Geometry: final body of the model. Coordinates: model frame, mm. A direction names the side the tool comes from. Coordinates: 2 decimals unless noted, no trailing zeros. Write each loop counter-clockwise with the first axis right and the second up, starting at its lowest first coordinate (ties: lowest second). Pieces come first, ordered by that corner, then holes. Notation, with made-up numbers: M 47,39.25 L 82,39.25 A17 ccw 82,71.25 Z; hole C 64,44 d1. An arc over 180 degrees is marked long. Write item = value, one per line. Start each with the question number.
Item 1: Pull-direction query (X, two-part tool) for faces 1 (the flat face through (-18.492, -4, 3)), 2 (the flat face through (25.4, -8, 3)), 3 (the cylindrical face through (12.532, -13.154, 3.026)), 4 (the flat face through (-24, -24.724, 3)); classes: +X half, -X half, draft (parallel to the pull), parting line (faces both ways), or undercut.
Item 2: Section B-B on y = 0.15. Output: boundary loops of the cut face in (x, z).
Item 3: Reachability of faces 5 (the flat face through (24, -5.84, 3)), 6 (the flat face through (-21, -1.039, 3)), 7 (the flat face through (-17.64, -19.01, 2.94)), 8 (the flat face through (-28, -10.437, 3)) from +Z, -Z, +X, -X, +Y, -Y: full face, straight path, thin tool, end or side. Return the list, or none.
Item 4: Section C-C on z = 0.9. Give the number of separate pieces and of enclosed holes in the cut face, plus the area to 3 significant figures.
Item 5: Section D-D on y = -17. Output: boundary loops of the cut face in (x, z).
Item 6: Ray query, L1, parallel to X at y = -1.5, z = 1.95 (3 decimals); L2, parallel to Y at x = -26, z = 1.85; L3, parallel to Y at x = 0.5, z = 2.6. Return the intervals inside material, ascending. Write a range as [from, to].
Item 7: First-contact query: pin 1 Ø1.4 at (y, z) = (-2, 1.5) entering from -X; pin 2 Ø3 at (y, z) = (-4, 4.5) entering from -X; pin 3 Ø0.6 at (x, z) = (-19, 2.5) entering from +Y. Flat tips, straight axial feed; report the tip coordinate or a pass-through.
Item 8: Section A-A on x = -1.5. Output: boundary loops of the cut face in (y, z).
from build123d import *

# Parameters (mm, degrees)
SKETCH1_W           = 12.3904
SKETCH1_H           = 13
BOSS_EXTRUDE1_DEPTH = 5.969
CUT_EXTRUDE1_DEPTH  = 41.286380146
SKETCH3_R           = 0.1984375
CUT_EXTRUDE2_DEPTH  = 41.286380146
FILLET1_R           = 3.175
FILLET2_R           = 1.5875
SKETCH4_W           = 12.7
SKETCH4_H           = 11.1125
CUT_EXTRUDE3_DEPTH  = 41.286380146
SKETCH5_W           = 10.16
SKETCH5_H           = 0.5
CUT_EXTRUDE4_DEPTH  = 41.286380146
FILLET8_R           = 0.1
CUT_EXTRUDE5_DEPTH  = 41.286380146
FILLET9_R           = 6.35


with BuildPart() as part:
    # Sketch1 → Boss-Extrude1 (new body)
    with BuildSketch(Plane.XY):
        Polygon((25.4, 2.263), (25.4, -10.437), (31.242, -10.437), (31.242, -23.137), (25.4, -23.137), (25.4, -24.7245), (22.225, -24.7245), (12.7, -12.85), (-12.7, -12.85), (-22.225, -24.7245), (-25.4, -24.7245), (-25.4, -23.137), (-31.242, -23.137), (-31.242, -10.437), (-25.4, -10.437), (-25.4, 2.263), (-31.242, 2.263), (-31.242, 14.963), (-25.4, 14.963), (-25.4, 18.138), (-22.225, 18.138), (-12.7, 12.85), (12.7, 12.85), (22.225, 18.138), (25.4, 18.138), (25.4, 14.963), (31.242, 14.963), (31.242, 2.263), align=None)
        Rectangle(SKETCH1_W, SKETCH1_H, mode=Mode.SUBTRACT)
    extrude(amount=BOSS_EXTRUDE1_DEPTH)

    # Sketch2 → Cut-Extrude1 (cut, through all)
    with BuildSketch(Plane.XY.offset(5.969)):
        Polygon((22.225, -2.3344), (22.225, -1.039), (19.05, -1.039), (19.05, -2.3344), (18.492, -2.3344), (18.492, -5.8396), (19.05, -5.8396), (19.05, -7.135), (22.225, -7.135), (22.225, -5.8396), (25.4, -5.8396), (25.4, -2.3344), align=None)
        Polygon((-19.05, -2.3344), (-19.05, -1.039), (-22.225, -1.039), (-22.225, -2.3344), (-25.4, -2.3344), (-25.4, -5.8396), (-22.225, -5.8396), (-22.225, -7.135), (-19.05, -7.135), (-19.05, -5.8396), (-18.492, -5.8396), (-18.492, -2.3344), align=None)
    extrude(amount=-CUT_EXTRUDE1_DEPTH, mode=Mode.SUBTRACT)

    # Sketch3 → Cut-Extrude2 (cut, through all)
    with BuildSketch(Plane.XY.offset(5.969)):
        with Locations((6.1952, 6.5)):
            Circle(SKETCH3_R)
        with Locations((-6.1952, 6.5)):
            Circle(SKETCH3_R)
        with Locations((-6.1952, -6.5)):
            Circle(SKETCH3_R)
        with Locations((6.1952, -6.5)):
            Circle(SKETCH3_R)
    extrude(amount=-CUT_EXTRUDE2_DEPTH, mode=Mode.SUBTRACT)

    # Fillet1
    fillet1_edges = [part.edges().sort_by_distance(p)[0] for p in [
        (12.7, -12.85, 2.9845),
        (-12.7, -12.85, 2.9845),
    ]]
    fillet(fillet1_edges, radius=FILLET1_R)

    # Fillet2
    fillet2_edges = [part.edges().sort_by_distance(p)[0] for p in [
        (22.225, -24.7245, 2.9845),
        (-22.225, -24.7245, 2.9845),
        (-22.225, 18.138, 2.9845),
        (22.225, 18.138, 2.9845),
    ]]
    fillet(fillet2_edges, radius=FILLET2_R)

    # Sketch4 → Cut-Extrude3 (cut, through all)
    with BuildSketch(Plane.XY.offset(5.969)):
        Rectangle(SKETCH4_W, SKETCH4_H)
    extrude(amount=-CUT_EXTRUDE3_DEPTH, mode=Mode.SUBTRACT)

    # Sketch5 → Cut-Extrude4 (cut, through all)
    with BuildSketch(Plane.XY.offset(5.969)):
        with Locations((0, 6.5)):
            Rectangle(SKETCH5_W, SKETCH5_H)
    extrude(amount=-CUT_EXTRUDE4_DEPTH, mode=Mode.SUBTRACT)

    # Fillet8
    fillet8_edges = [part.edges().sort_by_distance(p)[0] for p in [
        (5.08, 6.5, 2.9845),
        (-5.08, 6.5, 2.9845),
        (-5.08, 6.75, 2.9845),
        (5.08, 6.75, 2.9845),
    ]]
    fillet(fillet8_edges, radius=FILLET8_R)

    # Sketch6 → Cut-Extrude5 (cut, through all)
    with BuildSketch(Plane.XY.offset(5.969)):
        with BuildLine():
            Line((-15.7, 7.5), (-9.7, 7.5))
            ThreePointArc((-9.7, 7.5), (-8.7, 6.5), (-9.7, 5.5))
            Line((-9.7, 5.5), (-15.7, 5.5))
            ThreePointArc((-15.7, 5.5), (-16.7, 6.5), (-15.7, 7.5))
        make_face()
        with BuildLine():
            Line((-15.7, 1.15), (-9.7, 1.15))
            ThreePointArc((-9.7, 1.15), (-8.7, 0.15), (-9.7, -0.85))
            Line((-9.7, -0.85), (-15.7, -0.85))
            ThreePointArc((-15.7, -0.85), (-16.7, 0.15), (-15.7, 1.15))
        make_face()
    extrude(amount=-CUT_EXTRUDE5_DEPTH, mode=Mode.SUBTRACT)

    # Fillet9
    fillet9_edges = [part.edges().sort_by_distance(p)[0] for p in [
        (-12.7, 12.85, 2.9845),
        (12.7, 12.85, 2.9845),
    ]]
    fillet(fillet9_edges, radius=FILLET9_R)


solid = part.part
Responses:
q1.face_1 = -X half
q1.face_2 = +X half
q1.face_3 = undercut
q1.face_4 = draft
q2.outline = M -25.4,0 L -16.7,0 L -16.7,5.97 L -25.4,5.97 Z; M -8.7,0 L -6.35,0 L -6.35,5.97 L -8.7,5.97 Z; M 6.35,0 L 25.4,0 L 25.4,5.97 L 6.35,5.97 Z
q3.face_5 = +Z, -Z, +X
q3.face_6 = +Z, -Z
q3.face_7 = +Z, -Z, -Y
q3.face_8 = +Z, -Z, -X
q4.separate_pieces = 1
q4.enclosed_holes = 3
q4.area = 1,610 mm²
q5.outline = M -31.24,0 L -16.03,0 L -16.03,5.97 L -31.24,5.97 Z; M 16.03,0 L 31.24,0 L 31.24,5.97 L 16.03,5.97 Z
q6.L1 = [-25.4, -22.225], [-19.05, -6.35], [6.35, 19.05], [22.225, 25.4]
q6.L2 = [-23.14, -10.44], [2.26, 14.96]
q6.L3 = [-12.85, -6.5], [6.75, 12.85]
q7.pin_1 = -25.4
q7.pin_2 = -18.49
q7.pin_3 = 16.51
q8.outline = M -12.85,0 L -6.5,0 L -6.5,5.97 L -12.85,5.97 Z; M 6.75,0 L 12.85,0 L 12.85,5.97 L 6.75,5.97 Z
